Check sheet for the modelled part. Datum: model origin and axes. Units: mm. Face numbers are marked on the shaded views. A direction names the side the tool comes from. Give positions to 0.01 mm unless a question says otherwise; leave off trailing zeros. Order: outer loops, then holes, each group sorted by start corner. A loop starts at its lowest first (then second) coordinate and runs counter-clockwise, first axis right, second up.
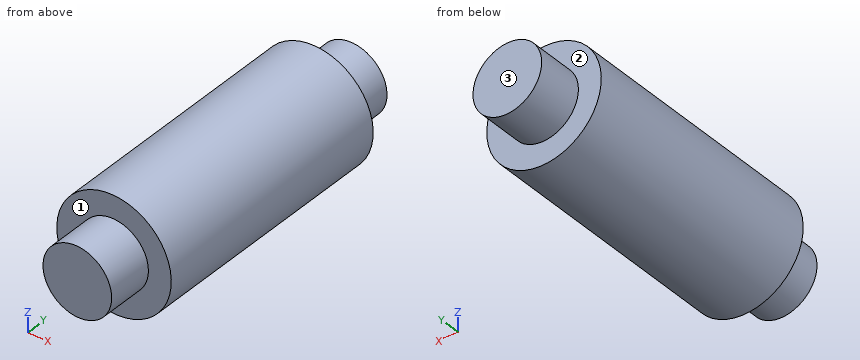
```python
from build123d import *

# Parameters (mm, degrees)
SKETCH_1_R      = 2.5
EXTRUDE_1_DEPTH = 11
SKETCH_2_R      = 1.5
EXTRUDE_2_DEPTH = 2
EXTRUDE_START   = 2
SKETCH_4_R      = 1.5
EXTRUDE_3_DEPTH = 2


with BuildPart() as part:
    # Эскиз1 → Бобышка-Вытянуть1 (new body)
    with BuildSketch(Plane(origin=(0, 0, 0), x_dir=(1, 0, 0), z_dir=(0, 1, 0))):
        with Locations(Location((0, 0, 0), (0, 0, 270))):
            Circle(SKETCH_1_R)
    extrude(amount=EXTRUDE_1_DEPTH)

    # Эскиз2 → Бобышка-Вытянуть2 (add)
    with BuildSketch(Plane(origin=(0, 11, 0), x_dir=(1, 0, 0), z_dir=(0, 1, 0))):
        with Locations(Location((0, 0, 0), (0, 0, 270))):
            Circle(SKETCH_2_R)
    extrude(amount=EXTRUDE_2_DEPTH)

    # Эскиз4 → Бобышка-Вытянуть3 (add)
    with BuildSketch(Plane.XZ.offset(EXTRUDE_START)):
        with Locations(Location((0, 0, 0), (0, 0, 90))):
            Circle(SKETCH_4_R)
    extrude(amount=-EXTRUDE_3_DEPTH)


solid = part.part
```
(1) Set-up check for the marked faces 1, 2 and 3: record each of +Z, -Z, +X, -X, +Y, -Y from which the full face is reachable in a straight line by a thin tool's end or side.
Response values:
face 1: -Y
face 2: +Y
face 3: +Z, -Z, +X, -X, +Y
(2) Cross-section at B-B on z = 0. Enter the section's corners in (x, y), then the cut area to 3 significant figures.
Response values:
outline: (-2.5, 0) - (-1.5, 0) - (-1.5, -2) - (1.5, -2) - (1.5, 0) - (2.5, 0) - (2.5, 11) - (1.5, 11) - (1.5, 13) - (-1.5, 13) - (-1.5, 11) - (-2.5, 11) - close
area: 67.0 mm2
(3) Material ranges on L1, parallel to Y at x = 0.3, z = 2.15; L2, parallel to X at y = 3, z = -0.5; L3, parallel to X at y = 2.75, z = 1.7, recorded low to high.
Response values:
L1: y = 0 to 11
L2: x = -2.45 to 2.45
L3: x = -1.83 to 1.83
(4) Cross-section at D-D on z = 1.85. Enter the section's corners in (x, y), then the cut area to 3 significant figures.
Response values:
outline: (-1.68, 0) - (1.68, 0) - (1.68, 11) - (-1.68, 11) - close
area: 37.0 mm2
(5) Cross-section at A-A on x = 0. Enter the section's corners in (y, z).
Response values:
outline: (-2, -1.5) - (0, -1.5) - (0, -2.5) - (11, -2.5) - (11, -1.5) - (13, -1.5) - (13, 1.5) - (11, 1.5) - (11, 2.5) - (0, 2.5) - (0, 1.5) - (-2, 1.5) - close
(6) Gauge pin test, flat ends, axial feed: pin 1 Ø2 at (y, z) = (6.5, 1.5) entering from -X; pin 2 Ø1 at (x, z) = (-2, 0.5) entering from +Y. Record the tip position at first contact, or that the pin passes through.
Response values:
pin 1: stops at x = -2.45
pin 2: stops at y = 11
(7) Cross-section at C-C on y = 2. Enter the section's corners in (x, z).
Response values:
outline: circle Ø5 at (0, 0)
